from build123d import *

# Parameters (mm, degrees)
SKETCH1_W           = 50
SKETCH1_H           = 50
BOSS_EXTRUDE1_DEPTH = 50
SKETCH2_W           = 50
SKETCH2_H           = 30
CUT_EXTRUDE1_DEPTH  = 5
SKETCH3_W           = 5
SKETCH3_H           = 30
BOSS_EXTRUDE2_DEPTH = 150
SKETCH4_R           = 35
BOSS_EXTRUDE3_DEPTH = 50
SKETCH5_OUTSIDE_W   = 287.05
SKETCH5_OUTSIDE_H   = 122.05
CUT_EXTRUDE2_DEPTH  = 60
SKETCH6_OUTSIDE_W   = 262.676
SKETCH6_OUTSIDE_H   = 98.214
CUT_EXTRUDE3_DEPTH  = 60
SKETCH7_R           = 5
CUT_EXTRUDE4_DEPTH  = 60
SKETCH8_OUTSIDE_W   = 262.676
SKETCH8_OUTSIDE_H   = 118.214
SKETCH8_OUTSIDE_R   = 23.965206127
CUT_EXTRUDE5_DEPTH  = 45
SKETCH9_OUTSIDE_W   = 262.676
SKETCH9_OUTSIDE_H   = 118.214
CUT_EXTRUDE6_DEPTH  = 47
CUT_EXTRUDE7_DEPTH  = 48.5


with BuildPart() as part:
    # Sketch1 → Boss-Extrude1 (new body)
    with BuildSketch(Plane.XY):
        with Locations((25, 25)):
            Rectangle(SKETCH1_W, SKETCH1_H)
    extrude(amount=BOSS_EXTRUDE1_DEPTH)

    # Sketch2 → Cut-Extrude1 (cut)
    with BuildSketch(Plane.XY.offset(50)):
        with Locations((25, 25)):
            Rectangle(SKETCH2_W, SKETCH2_H)
    extrude(amount=-CUT_EXTRUDE1_DEPTH, mode=Mode.SUBTRACT)

    # Sketch3 → Boss-Extrude2 (add)
    with BuildSketch(Plane(origin=(50, 0, 0), x_dir=(0, 0, -1), z_dir=(1, 0, 0))):
        with Locations((-2.5, 25)):
            Rectangle(SKETCH3_W, SKETCH3_H)
    extrude(amount=BOSS_EXTRUDE2_DEPTH)

    # Sketch4 → Boss-Extrude3 (add)
    with BuildSketch(Plane(origin=(0, 0, 0), x_dir=(-1, 0, 0), z_dir=(0, 0, -1))):
        with Locations((-200, 25)):
            Circle(SKETCH4_R)
    extrude(amount=-BOSS_EXTRUDE3_DEPTH)

    # Sketch5 outside → Cut-Extrude2 (cut)
    with BuildSketch(Plane(origin=(0, 0, 0), x_dir=(-1, 0, 0), z_dir=(0, 0, -1))):
        with Locations((-117.5, 25)):
            Rectangle(SKETCH5_OUTSIDE_W, SKETCH5_OUTSIDE_H)
        with BuildLine():
            Line((-50, 40), (-35.53775066, 40))
            ThreePointArc((-35.53775066, 40), (-20.53775066, 25), (-35.53775066, 10))
            Line((-35.53775066, 10), (-50, 10))
            Line((-50, 10), (-247.49593965, -30.086255952))
            Line((-247.49593965, -30.086255952), (-247.49593965, 85.804552417))
            Line((-247.49593965, 85.804552417), (-50, 40))
        make_face(mode=Mode.SUBTRACT)
    extrude(amount=-CUT_EXTRUDE2_DEPTH, mode=Mode.SUBTRACT)

    # Sketch6 outside → Cut-Extrude3 (cut)
    with BuildSketch(Plane(origin=(0, 40, 0), x_dir=(1, 0, 0), z_dir=(0, 1, 0))):
        with Locations((127.769, -25)):
            Rectangle(SKETCH6_OUTSIDE_W, SKETCH6_OUTSIDE_H)
        Polygon((50, -5), (20.53775066, -5), (20.53775066, 0), (245.971060593, 0), (245.971060593, -81.039305363), (133.254405627, -81.039305363), align=None, mode=Mode.SUBTRACT)
    extrude(amount=-CUT_EXTRUDE3_DEPTH, mode=Mode.SUBTRACT)

    # Sketch7 → Cut-Extrude4 (cut)
    with BuildSketch(Plane.XY.offset(50)):
        with Locations((200, 25)):
            Circle(SKETCH7_R)
    extrude(amount=-CUT_EXTRUDE4_DEPTH, mode=Mode.SUBTRACT)

    # Sketch8 outside → Cut-Extrude5 (cut)
    with BuildSketch(Plane.XY.offset(50)):
        with Locations((127.769, 25)):
            Rectangle(SKETCH8_OUTSIDE_W, SKETCH8_OUTSIDE_H)
        with Locations((200, 25)):
            Circle(SKETCH8_OUTSIDE_R, mode=Mode.SUBTRACT)
    extrude(amount=-CUT_EXTRUDE5_DEPTH, mode=Mode.SUBTRACT)

    # Sketch9 outside → Cut-Extrude6 (cut)
    with BuildSketch(Plane.XY.offset(5)):
        with Locations((127.769, 25)):
            Rectangle(SKETCH9_OUTSIDE_W, SKETCH9_OUTSIDE_H)
        with BuildLine():
            Line((168.377223398, 40), (181.309598594, 40))
            ThreePointArc((181.309598594, 40), (223.965206127, 25), (181.309598594, 10))
            Line((181.309598594, 10), (168.377223398, 10))
            Line((168.377223398, 10), (164.401061703, 1.034793873))
            Line((164.401061703, 1.034793873), (16.874562841, 1.034793873))
            Line((16.874562841, 1.034793873), (16.874562841, 40))
            Line((16.874562841, 40), (168.377223398, 40))
        make_face(mode=Mode.SUBTRACT)
    extrude(amount=-CUT_EXTRUDE6_DEPTH, mode=Mode.SUBTRACT)

    # Sketch10 → Cut-Extrude7 (cut, symmetric)
    with BuildSketch(Plane(origin=(0, 40, 0), x_dir=(1, 0, 0), z_dir=(0, 1, 0))):
        Polygon((232.409731391, -29.094811743), (165.185777122, -29.094811743), (165.185777122, -67.022723685), (235.548593069, -67.022723685), align=None)
    extrude(amount=CUT_EXTRUDE7_DEPTH, both=True, mode=Mode.SUBTRACT)


solid = part.part
Here's how the part is built. I have some questions about the finished solid (model axes, mm). A direction names the side the tool comes from. Coordinates: 2 decimals unless noted, no trailing zeros. Write each loop counter-clockwise with the first axis right and the second up, starting at its lowest first coordinate (ties: lowest second). Pieces come first, ordered by that corner, then holes.
1) If I drill on line 1 (Y direction, x = 200, z = 10); line 2 (Z direction, x = 173.5, y = 26); line 3 (X direction, y = 29.5, z = 15), over which ranges is the centre line in solid material (lowest first)?
Filled in:
line 1: y = 1.03 to 20, 30 to 48.97
line 2: z = 0 to 5
line 3: x = 176.46 to 197.82, 202.18 to 223.54
2) If we section it at C-C (z = 2.75): List the corners of the cut face in (x, y) for me.
Filled in:
outline: (35.54, 10) - (181.31, 10) arc R23.97 ccw (long way) to (181.31, 40) - (35.54, 40) arc R15 ccw to start; hole circle Ø10 at (200, 25)
3) I'm going to push flat-ended pins straight in: pin 1 (3 mm diameter, centred on y = 13.5, z = 22, fed in from -X); pin 2 (6 mm diameter, centred on x = 42.5, y = 13, fed in from +Z); pin 3 (6 mm diameter, centred on y = 43.5, z = 15.5, fed in from +X). Where does each tip first touch, or does it pass through?
Filled in:
pin 1: stops at x = 178.22
pin 2: stops at z = 5
pin 3: stops at x = 218.28
4) Which directions (+Z, -Z, +X, -X, +Y, -Y) give clear straight access to the entire face, cutting with the end or side of a thin tool? Please do faces 4 (the face through (107, 10, 2)), 5 (the face through (121, 25, 0)), 6 (the face through (109, 40, 2)).
Filled in:
face 4: +Z, -Z, -X, -Y
face 5: -Z, +X, -X, +Y, -Y
face 6: +Z, -Z, -X, +Y
5) Thinking about a two-plate mould opening in Y: for faces 1 (the face through (102, 25, 5)), 2 (the face through (202.307, 20.564, 14.751)), 3 (the face through (20.54, 25.33, 2.46)), which applies, +Y half, -Y half, draft (parallel to the pull), parting line (faces both ways), or undercut?
Filled in:
face 1: draft
face 2: undercut
face 3: parting line
6) If we section it at B-B (y = 25): List the corners of the cut face in (x, z) for me, plus the area to 3 significant figures.
Filled in:
outline: (20.54, 0) - (195, 0) - (195, 29.09) - (176.03, 29.09) - (176.03, 5) - (20.54, 5) - close; (205, 0) - (223.97, 0) - (223.97, 29.09) - (205, 29.09) - close
area: 1,880 mm2
7) If we section it at D-D (x = 100): List the corners of the cut face in (y, z) for me.
Filled in:
outline: (10, 0) - (40, 0) - (40, 5) - (10, 5) - close
8) If we section it at A-A (x = 200): List the corners of the cut face in (y, z) for me.
Filled in:
outline: (1.03, 0) - (20, 0) - (20, 29.09) - (1.03, 29.09) - close; (30, 0) - (48.97, 0) - (48.97, 29.09) - (30, 29.09) - close
